from build123d import *

# Parameters (mm, degrees)
SKETCH_1_R               = 22
EXTRUDE_1_DEPTH          = 2
SKETCH_3_R               = 1.25
CUT_EXTRUDE_1_DEPTH      = 3
SKETCH_4_R               = 3.5
CUT_EXTRUDE_2_DEPTH      = 3
SKETCH_6_R               = 3
EXTRUDE_3_DEPTH          = 9.5
SKETCH_8_R               = 1
CUT_EXTRUDE_4_DEPTH      = 11.5
CUT_EXTRUDE_3_DEPTH      = 6
PATTERN_CIRCULAR_1_COUNT = 4
FILLET_2_R               = 1.5
FILLET_3_R               = 1.5


with BuildPart() as part:
    # 草图1 → 凸台-拉伸1 (new body)
    with BuildSketch(Plane.XY):
        Circle(SKETCH_1_R)
    extrude(amount=EXTRUDE_1_DEPTH)

    # 草图3 → 切除-拉伸1 (cut)
    with BuildSketch(Plane(origin=(0, 0, 0), x_dir=(-1, 0, 0), z_dir=(0, 0, -1))):
        with Locations((6, 0)):
            Circle(SKETCH_3_R)
    cut_extrude_1 = extrude(amount=-CUT_EXTRUDE_1_DEPTH, mode=Mode.SUBTRACT)

    # 草图4 → 切除-拉伸2 (cut)
    with BuildSketch(Plane(origin=(0, 0, 0), x_dir=(-1, 0, 0), z_dir=(0, 0, -1))):
        Circle(SKETCH_4_R)
    extrude(amount=-CUT_EXTRUDE_2_DEPTH, mode=Mode.SUBTRACT)

    # 草图6 → 凸台-拉伸3 (add)
    with BuildSketch(Plane(origin=(0, 0, 0), x_dir=(-1, 0, 0), z_dir=(0, 0, -1))):
        with Locations((0, -19)):
            Circle(SKETCH_6_R)
    extrude_3 = extrude(amount=EXTRUDE_3_DEPTH)

    # 草图8 → 切除-拉伸4 (cut)
    with BuildSketch(Plane(origin=(0, 0, -9.5), x_dir=(-1, 0, 0), z_dir=(0, 0, -1))):
        with Locations((0, -19)):
            Circle(SKETCH_8_R)
    cut_extrude_4 = extrude(amount=-CUT_EXTRUDE_4_DEPTH, mode=Mode.SUBTRACT)

    # 草图7 → 切除-拉伸3 (cut)
    with BuildSketch(Plane(origin=(0, 0, 0), x_dir=(-1, 0, 0), z_dir=(0, 0, -1))):
        Polygon((-1.961261338, 7.845045353), (-7.845045353, 1.961261338), (-30.512752563, 7.628188141), (-7.628188141, 30.512752563), align=None)
    cut_extrude_3 = extrude(amount=-CUT_EXTRUDE_3_DEPTH, mode=Mode.SUBTRACT)

    # 阵列(圆周)1: 切除-拉伸1, 凸台-拉伸3, 切除-拉伸4, 切除-拉伸3 ×4 about axis
    pattern_circular_1_axis = Axis((0, 0, 0), (0, 0, 1))
    for i in range(1, PATTERN_CIRCULAR_1_COUNT):
        add(cut_extrude_1.rotate(pattern_circular_1_axis, i * 360 / PATTERN_CIRCULAR_1_COUNT), mode=Mode.SUBTRACT)
        add(extrude_3.rotate(pattern_circular_1_axis, i * 360 / PATTERN_CIRCULAR_1_COUNT))
        add(cut_extrude_4.rotate(pattern_circular_1_axis, i * 360 / PATTERN_CIRCULAR_1_COUNT), mode=Mode.SUBTRACT)
        add(cut_extrude_3.rotate(pattern_circular_1_axis, i * 360 / PATTERN_CIRCULAR_1_COUNT), mode=Mode.SUBTRACT)

    # 圆角2
    fillet_2_edges = [part.edges().sort_by_distance(p)[0] for p in [
        (-5.335783751, -21.343135003, 1),
        (-21.343135003, -5.335783751, 1),
        (21.343135003, -5.335783751, 1),
        (5.335783751, -21.343135003, 1),
        (5.335783751, 21.343135003, 1),
        (21.343135003, 5.335783751, 1),
        (-21.343135003, 5.335783751, 1),
        (-5.335783751, 21.343135003, 1),
    ]]
    fillet(fillet_2_edges, radius=FILLET_2_R)

    # 圆角3
    fillet_3_edges = [part.edges().sort_by_distance(p)[0] for p in [
        (-7.845045353, -1.961261338, 1),
        (-1.961261338, -7.845045353, 1),
        (1.961261338, -7.845045353, 1),
        (7.845045353, -1.961261338, 1),
        (7.845045353, 1.961261338, 1),
        (1.961261338, 7.845045353, 1),
        (-1.961261338, 7.845045353, 1),
        (-7.845045353, 1.961261338, 1),
    ]]
    fillet(fillet_3_edges, radius=FILLET_3_R)


solid = part.part
For this review, take the finished solid that the model builds, in its own axes (mm). A direction names the side the tool comes from. Give positions to 0.01 mm unless a question says otherwise; leave off trailing zeros. Loops run counter-clockwise (first coordinate to the right, second up) from the corner with the lowest first, then second, coordinate; pieces in that order, holes last. Notation, with made-up numbers: (66, -13) - (118, -13) arc R32 cw to (118, 13) - close; hole circle Ø8 at (2, 79.25). An arc over 180 degrees is marked (long way). Write each question's results on one line, items separated by ' | '.
(1) For faces 1 (the flat face through (-3.543, 14.174, 0.986)), 2 (the flat face through (-14.174, -3.543, 0.986)), 3 (the flat face through (4.87, 4.936, 0.986)), 4 (the flat face through (-1, 18, -9.5)), list the 3-axis set-ups (+Z, -Z, +X, -X, +Y, -Y) from which the entire face can be reached by the end or side of a thin tool; tool diameter is ignored.
Conclusion:
face 1: +Z, -Z, -X | face 2: +Z, -Z, -Y | face 3: +Z, -Z | face 4: -Z, +X, -X, +Y, -Y
(2) For pin 1 Ø3 at (x, y) = (0, 6) entering from -Z, flat-tipped, find the tip position at first contact; note if it passes through.
Conclusion:
pin 1: z = 0
(3) Draft analysis for pull direction Y (two halves, no side actions). For faces 5 (the flat face through (18, 1, -9.5)), 6 (the cylindrical face through (-21.93, -0.65, -4.68)), 7 (the flat face through (-4.936, 4.87, 0.986)), 8 (the cylindrical face through (21.03, -4.75, 0.99)), state which applies: +Y half, -Y half, draft (parallel to the pull), parting line (faces both ways), or undercut.
Conclusion:
face 5: draft | face 6: parting line | face 7: undercut | face 8: -Y half
(4) Take a section at B-B (x = 19). Give the boundary of the cut face in (y, z), then the cut area to 3 significant figures.
Conclusion:
outline: (-4.75, 0) - (-3, 0) - (-3, -9.5) - (-1, -9.5) - (-1, 2) - (-4.75, 2) - close; (1, -9.5) - (3, -9.5) - (3, 0) - (4.75, 0) - (4.75, 2) - (1, 2) - close | area: 53.0 mm^2
(5) Take a section at A-A (z = -2.5). Give the boundary of the cut face in (x, y).
Conclusion:
outline: circle Ø6 at (-19, 0); circle Ø6 at (0, -19); circle Ø6 at (0, 19); circle Ø6 at (19, 0); hole circle Ø2 at (-19, 0); hole circle Ø2 at (0, -19); hole circle Ø2 at (0, 19); hole circle Ø2 at (19, 0)
(6) For line 1 along Y through (x, z) = (0, -3); line 2 along Z through (x, y) = (-8, -0.5), list the stretches that pass through material, from the lowest coordinate up.
Conclusion:
line 1: -22 to -20, -18 to -16, 16 to 18, 20 to 22 | line 2: 0 to 2
(7) Take a section at D-D (x = -12). Give the boundary of the cut face in (y, z), then the cut area to 3 significant figures.
Conclusion:
outline: (-3, 0) - (3, 0) - (3, 2) - (-3, 2) - close | area: 12.0 mm^2
(8) Take a section at C-C (y = 6). Give the boundary of the cut face in (x, z), then the cut area to 3 significant figures.
Conclusion:
outline: (-3.81, 0) - (-1.25, 0) - (-1.25, 2) - (-3.81, 2) - close; (1.25, 0) - (3.81, 0) - (3.81, 2) - (1.25, 2) - close | area: 10.2 mm^2
